Source: CAD feature listing. Evaluate the final solid. Frame: model axes, mm. Give positions to 0.01 mm unless a question says otherwise; leave off trailing zeros. Write each loop counter-clockwise with the first axis right and the second up, starting at its lowest first coordinate (ties: lowest second). Pieces come first, ordered by that corner, then holes. Notation, with made-up numbers: (28, 24) -> (66, 24) arc R11 ccw to (66, 41) -> close; hole circle Ø7 at (22.5, 72.25). An arc over 180 degrees is marked (long way). Write item = value, one per line.
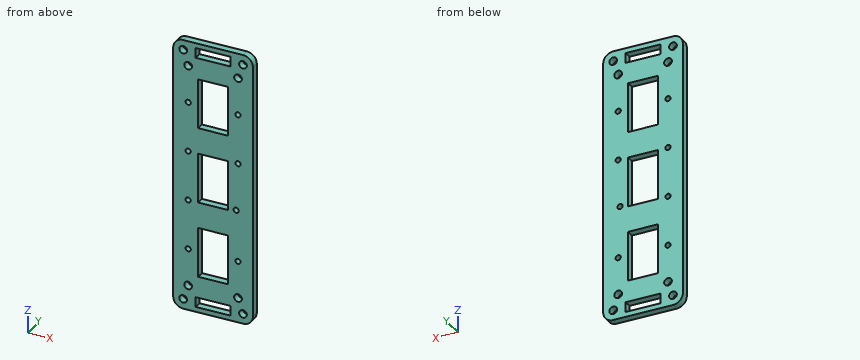
from build123d import *

# Parameters (mm, degrees)
SKETCH_1_R      = 1.05
SKETCH_1_R_2    = 1.55
SKETCH_1_W      = 12
SKETCH_1_H      = 20
SKETCH_1_W_2    = 14
SKETCH_1_H_2    = 4
EXTRUDE_1_DEPTH = 3


with BuildPart() as part:
    # 草图1 → 凸台-拉伸1 (new body)
    with BuildSketch(Plane(origin=(0, 0, 0), x_dir=(1, 0, 0), z_dir=(0, 1, 0))):
        with BuildLine():
            Line((-16, -37.476129922), (-16, -51))
            ThreePointArc((-16, -51), (-14.828427125, -53.828427125), (-12, -55))
            Line((-12, -55), (12, -55))
            ThreePointArc((12, -55), (14.828427125, -53.828427125), (16, -51))
            Line((16, -51), (16, -37.476129922))
            Line((16, -37.476129922), (16, 25.467140075))
            Line((16, 25.467140075), (16, 51))
            ThreePointArc((16, 51), (14.828427125, 53.828427125), (12, 55))
            Line((12, 55), (-12, 55))
            ThreePointArc((-12, 55), (-14.828427125, 53.828427125), (-16, 51))
            Line((-16, 51), (-16, 31.142350414))
            Line((-16, 31.142350414), (-16, -37.476129922))
        make_face()
        with Locations(Location((-10, 30, 0), (0, 0, 270))):
            Circle(SKETCH_1_R, mode=Mode.SUBTRACT)
        with Locations(Location((10, 30, 0), (0, 0, 270))):
            Circle(SKETCH_1_R, mode=Mode.SUBTRACT)
        with Locations(Location((-10, 10, 0), (0, 0, 270))):
            Circle(SKETCH_1_R, mode=Mode.SUBTRACT)
        with Locations(Location((10, -10, 0), (0, 0, 270))):
            Circle(SKETCH_1_R, mode=Mode.SUBTRACT)
        with Locations(Location((-10, -30, 0), (0, 0, 270))):
            Circle(SKETCH_1_R, mode=Mode.SUBTRACT)
        with Locations(Location((10, -30, 0), (0, 0, 270))):
            Circle(SKETCH_1_R, mode=Mode.SUBTRACT)
        with Locations(Location((10, -45, 0), (0, 0, 270))):
            Circle(SKETCH_1_R_2, mode=Mode.SUBTRACT)
        with Locations(Location((-10, -45, 0), (0, 0, 270))):
            Circle(SKETCH_1_R_2, mode=Mode.SUBTRACT)
        with Locations(Location((10, 45, 0), (0, 0, 270))):
            Circle(SKETCH_1_R_2, mode=Mode.SUBTRACT)
        with Locations(Location((-10, 45, 0), (0, 0, 270))):
            Circle(SKETCH_1_R_2, mode=Mode.SUBTRACT)
        with Locations(Location((9.25753788, 9.25753788, 0), (0, 0, 270))):
            Circle(SKETCH_1_R, mode=Mode.SUBTRACT)
        with Locations(Location((-10, -10, 0), (0, 0, 270))):
            Circle(SKETCH_1_R, mode=Mode.SUBTRACT)
        with Locations(Location((-12, 51, 0), (0, 0, 270))):
            Circle(SKETCH_1_R_2, mode=Mode.SUBTRACT)
        with Locations(Location((12, 51, 0), (0, 0, 270))):
            Circle(SKETCH_1_R_2, mode=Mode.SUBTRACT)
        with Locations(Location((-12, -51, 0), (0, 0, 270))):
            Circle(SKETCH_1_R_2, mode=Mode.SUBTRACT)
        with Locations(Location((12, -51, 0), (0, 0, 270))):
            Circle(SKETCH_1_R_2, mode=Mode.SUBTRACT)
        with Locations((0, 30.422470983)):
            Rectangle(SKETCH_1_W, SKETCH_1_H, mode=Mode.SUBTRACT)
        with Locations((0, 51)):
            Rectangle(SKETCH_1_W_2, SKETCH_1_H_2, mode=Mode.SUBTRACT)
        with Locations((0, -30.422470983)):
            Rectangle(SKETCH_1_W, SKETCH_1_H, mode=Mode.SUBTRACT)
        with Locations((0, -51)):
            Rectangle(SKETCH_1_W_2, SKETCH_1_H_2, mode=Mode.SUBTRACT)
        Rectangle(SKETCH_1_W, SKETCH_1_H, mode=Mode.SUBTRACT)
    extrude(amount=EXTRUDE_1_DEPTH)


solid = part.part
1) Cut plane C-C (z = -45). Return the cut outline in (x, y).
Computed:
outline = (-16, 0) -> (-11.55, 0) -> (-11.55, 3) -> (-16, 3) -> close; (-8.45, 0) -> (8.45, 0) -> (8.45, 3) -> (-8.45, 3) -> close; (11.55, 0) -> (16, 0) -> (16, 3) -> (11.55, 3) -> close
2) Cut plane B-B (x = -4.5). Return the cut outline in (y, z), then the cut area to 3 significant figures.
Computed:
outline = (0, -55) -> (3, -55) -> (3, -53) -> (0, -53) -> close; (0, -49) -> (3, -49) -> (3, -40.42) -> (0, -40.42) -> close; (0, -20.42) -> (3, -20.42) -> (3, -10) -> (0, -10) -> close; (0, 10) -> (3, 10) -> (3, 20.42) -> (0, 20.42) -> close; (0, 40.42) -> (3, 40.42) -> (3, 49) -> (0, 49) -> close; (0, 53) -> (3, 53) -> (3, 55) -> (0, 55) -> close
area = 126 mm²
3) Cut plane A-A (z = 5.5). Return the cut outline in (x, y).
Computed:
outline = (-16, 0) -> (-6, 0) -> (-6, 3) -> (-16, 3) -> close; (6, 0) -> (16, 0) -> (16, 3) -> (6, 3) -> close
4) Material intervals for L1, parallel to X at y = 1.2, z = -51; L2, parallel to Z at x = -6.5, y = 1.95; L3, parallel to Z at x = -2.5, y = 1.05, sorted ascending.
Computed:
L1 = -16 to -13.55, -10.45 to -7, 7 to 10.45, 13.55 to 16
L2 = -55 to -53, -49 to 49, 53 to 55
L3 = -55 to -53, -49 to -40.42, -20.42 to -10, 10 to 20.42, 40.42 to 49, 53 to 55
5) Cut plane D-D (y = 1.4). State how many separate pieces and enclosed holes the cut face has, then the cut area to 3 significant figures.
Computed:
separate_pieces = 1
enclosed_holes = 21
area = 2,590 mm²
6) Contact query for flat-ended pins moving along their axis: pin 1 (2.5 mm diameter, centred on x = -10, z = -30, fed in from +Y); pin 2 (1.7 mm diameter, centred on x = 10, z = 30, fed in from -Y) (3 decimals). Output: stop coordinate, or through.
Computed:
pin_1 = 3
pin_2 = through
